Geometry: final body of the model. Coordinates: model frame, mm. A direction names the side the tool comes from. Give positions to 0.01 mm unless a question says otherwise; leave off trailing zeros. Write each loop counter-clockwise with the first axis right and the second up, starting at its lowest first coordinate (ties: lowest second). Pieces come first, ordered by that corner, then holes. Notation, with made-up numbers: M -3,27.5 L 25,27.5 A13 ccw 25,39.5 Z; hole C 40.5,-12.75 d11. An arc over 180 degrees is marked long. Use one line per item in the form item = value. Start each with the question number.
Item 1: Access query for faces 5 (the flat face through (155.834, 2.88, 20.054)), 6 (the flat face through (57, 3, 0)), 7 (the flat face through (6.89, 2.88, 173.08)), 8 (the flat face through (171, 3, 0)), 9 (the flat face through (6, 3, 0)). Directions: +Z, -Z, +X, -X, +Y, -Y. A direction counts if a zero-diameter tool reaches every point of the face in a straight line with its end or side. Return the directions, or none.
Item 2: Contact query for flat-ended pins moving along their axis: P1, Ø2, axis at y = 5, z = 80, coming from the +X side; P2, Ø1.8, axis at y = 1.5, z = -2, coming from the +X side; P3, Ø1.8, axis at x = 61, y = 3, coming from the -Z side; P4, Ø1, axis at y = 2.5, z = 94.5, coming from the -X side. Output: stop coordinate, or through.
Item 3: Section query B-B on z = 123. Return loops of the section in (x, y), then the cut area to 3 significant figures.
Item 4: Section query C-C on x = 110.5. Return loops of the section in (y, z).
Item 5: Material intervals for line 1 along Z through (x, y) = (108, 1.05); line 2 along Z through (x, y) = (8, 4.5); line 3 along X through (y, z) = (2.15, 168), sorted ascending. Write a range as from..to.
Item 6: Section query A-A on y = 4.5. Return loops of the section in (x, z).
Item 7: Pull-direction query (X, two-part tool) for faces 1 (the flat face through (152, 3, -5.842)), 2 (the flat face through (126.78, 2.88, 57.37)), 3 (the flat face through (101.6, 3, -3)), 4 (the flat face through (166.78, 2.88, 13.29)); classes: released by +X, released by -X, zero draft, split by the parting line, or undercut.
from build123d import *

# Parameters (mm, degrees)
F0_W     = 25.4
F0_H     = 5.842
F1_DEPTH = 5.842


with BuildPart() as f1:
    # F0 (on Front) → F1 (new body)
    with BuildSketch(Plane.XZ):
        Polygon((8.980256, 175.169744), (0, 184.15), (0, 0), (12.7, 0), (38.1, 0), (76.2, 0), (101.6, 0), (139.7, 0), (165.1, 0), (177.8, 0), (177.8, 6.35), (168.819744, 15.330256), (164.688826, 11.199338), (146.728314, 29.159851), (150.859232, 33.290768), (102.011174, 82.138826), (97.880256, 78.007908), (79.919744, 95.96842), (84.050662, 100.099338), (26.940768, 157.209232), (22.809851, 153.078314), (4.849338, 171.038826), align=None)
        with Locations((25.4, -2.921)):
            Rectangle(F0_W, F0_H)
        with Locations((152.4, -2.921)):
            Rectangle(F0_W, F0_H)
        with Locations((88.9, -2.921)):
            Rectangle(F0_W, F0_H)
    extrude(amount=-F1_DEPTH)


solid = f1.part
Answer sheet:
q1.face_5 = +Y, -Y
q1.face_6 = -Z, +Y, -Y
q1.face_7 = +X, +Y, -Y
q1.face_8 = -Z, +X, +Y, -Y
q1.face_9 = -Z, -X, +Y, -Y
q2.P1 = 105.15
q2.P2 = 165.1
q2.P3 = 0
q2.P4 = 0
q3.outline = M 0,0 L 61.15,0 L 61.15,5.84 L 0,5.84 Z
q3.area = 357 mm2
q4.outline = M 0,0 L 5.84,0 L 5.84,73.65 L 0,73.65 Z
q5.line_1 = 0..76.15
q5.line_2 = 0..167.89, 174.19..176.15
q5.line_3 = 0..7.89
q6.outline = M 0,0 L 12.7,0 L 12.7,-5.84 L 38.1,-5.84 L 38.1,0 L 76.2,0 L 76.2,-5.84 L 101.6,-5.84 L 101.6,0 L 139.7,0 L 139.7,-5.84 L 165.1,-5.84 L 165.1,0 L 177.8,0 L 177.8,6.35 L 168.82,15.33 L 164.69,11.2 L 146.73,29.16 L 150.86,33.29 L 102.01,82.14 L 97.88,78.01 L 79.92,95.97 L 84.05,100.1 L 26.94,157.21 L 22.81,153.08 L 4.85,171.04 L 8.98,175.17 L 0,184.15 Z
q7.face_1 = zero draft
q7.face_2 = released by +X
q7.face_3 = undercut
q7.face_4 = undercut
